from build123d import *

# Parameters (mm, degrees)
BOSS_EXTRUDE10_DEPTH = 1
BOSS_EXTRUDE11_DEPTH = 2
FILLET1_R            = 1
SKETCH22_R           = 1.6
CUT_EXTRUDE1_DEPTH   = 10


with BuildPart() as part:
    # Sketch20 → Boss-Extrude10 (new body)
    with BuildSketch(Plane(origin=(0, 0, 0), x_dir=(1, 0, 0), z_dir=(0, 1, 0))):
        with BuildLine():
            Line((-28, 14.425), (-20.5, 14.425))
            Line((-20.5, 14.425), (-20.5, 13.245))
            Line((-20.5, 13.245), (20.5, 13.245))
            Line((20.5, 13.245), (20.5, 14.425))
            Line((20.5, 14.425), (28, 14.425))
            ThreePointArc((28, 14.425), (28.707106781, 14.132106781), (29, 13.425))
            Line((29, 13.425), (29, -13.425))
            ThreePointArc((29, -13.425), (28.707106781, -14.132106781), (28, -14.425))
            Line((28, -14.425), (20.5, -14.425))
            Line((20.5, -14.425), (20.5, -13.245))
            Line((20.5, -13.245), (-20.5, -13.245))
            Line((-20.5, -13.245), (-20.5, -14.425))
            Line((-20.5, -14.425), (-28, -14.425))
            ThreePointArc((-28, -14.425), (-28.707106781, -14.132106781), (-29, -13.425))
            Line((-29, -13.425), (-29, 13.425))
            ThreePointArc((-29, 13.425), (-28.707106781, 14.132106781), (-28, 14.425))
        make_face()
    extrude(amount=BOSS_EXTRUDE10_DEPTH)

    # Sketch21 → Boss-Extrude11 (add)
    with BuildSketch(Plane.XZ):
        Polygon((-27.825, 3.25), (-26.825, 3.25), (-26.825, -12.25), (16.5, -12.25), (16.5, -13.25), (-27.825, -13.25), align=None)
        Polygon((-17.825, 13.25), (-17.825, 12.25), (26.825, 12.25), (26.825, 0), (27.825, 0), (27.825, 13.25), align=None)
    extrude(amount=BOSS_EXTRUDE11_DEPTH)

    # Fillet1
    fillet1_edges = [part.edges().sort_by_distance(p)[0] for p in [
        (-20.5, 0, -13.8375),
        (20.5, 0, -13.835),
        (20.5, 0, 13.8375),
        (-20.5, 0, 13.835),
    ]]
    fillet(fillet1_edges, radius=FILLET1_R - 0.0001)  # a hair under: the kernel refuses the full size

    # Sketch22 → Cut-Extrude1 (cut)
    with BuildSketch(Plane.XZ):
        with Locations(Location((-24.627459856, 9.750471763, 0), (0, 0, 270))):
            Circle(SKETCH22_R)
    extrude(amount=-CUT_EXTRUDE1_DEPTH, mode=Mode.SUBTRACT)


solid = part.part
Can you work these out from the model? Positions are in its coordinate system, mm. A direction names the side the tool comes from. Give positions to 0.01 mm unless a question says otherwise; leave off trailing zeros. Write each loop counter-clockwise with the first axis right and the second up, starting at its lowest first coordinate (ties: lowest second). Pieces come first, ordered by that corner, then holes. Notation, with made-up numbers: M -20,1.5 L 8,1.5 A29 cw 8,28.5 Z; hole C -12,60.5 d6. An arc over 180 degrees is marked long. Answer in a Markdown table with one row per item. Add a question column.
Item 1: We'd pull the mould along X, two halves only. Please class faces 1 (the flat face through (27.825, -1, 7)), 2 (the flat face through (-12, -2, -13)), 3 (the cylindrical face through (20.801, 0.285, -13.843)): released by +X, released by -X, zero draft, split by the parting line, or undercut.
Item 2: Please list where these lines run through material, in increasing order: L1, parallel to Z at x = -6, y = -0.75; L2, parallel to Y at x = 26, z = -1.75; L3, parallel to Z at x = 24, y = -1.65.
Item 3: Imagine slicing it at A-A, the plane y = -0.9. Write out the boundary of the cut face in (x, z) (3 decimals).
Item 4: Imagine slicing it at C-C, the plane x = -4. Write out the boundary of the cut face in (y, z) (3 decimals).
Item 5: Imagine slicing it at D-D, the plane z = 5.25. Write out the boundary of the cut face in (x, y) (3 decimals), plus the area to 3 significant figures.
Item 6: For pin 1 Ø1 at (x, y) = (-6.5, -0.5) entering from +Z; pin 2 Ø1.6 at (y, z) = (-1, -3.5) entering from -X (3 decimals); pin 3 Ø0.8 at (x, y) = (6, 0.5) entering from -Z (3 decimals), each with a flat end and sliding along its axis, tell me the tip position at first contact or that it passes through.
Item 7: Imagine slicing it at B-B, the plane z = 8.75. Write out the boundary of the cut face in (x, y) (3 decimals).
Item 8: On a 3-axis mill with a long thin cutter (end or side, diameter ignored), from which of +Z, -Z, +X, -X, +Y, -Y can I reach the whole of each face in a straight line? I mean faces 4 (the cylindrical face through (-20.801, 0.285, 13.843)), 5 (the flat face through (-17.825, -1, 13)), 6 (the flat face through (4, -1, 12.25)), 7 (the flat face through (16.5, -1, -13)). Say none if no direction works.
Evaluation:
| question | item | result |
|---|---|---|
| 1 | face 1 | released by +X |
| 1 | face 2 | zero draft |
| 1 | face 3 | undercut |
| 2 | L1 | z = -13.25 to -12.25, 12.25 to 13.25 |
| 2 | L2 | y = 0 to 1 |
| 2 | L3 | z = 12.25 to 13.25 |
| 3 | outline | M -27.825,-13.25 L 16.5,-13.25 L 16.5,-12.25 L -26.825,-12.25 L -26.825,3.25 L -27.825,3.25 Z; M -17.825,12.25 L 26.825,12.25 L 26.825,0 L 27.825,0 L 27.825,13.25 L -17.825,13.25 Z |
| 4 | outline | M -2,-13.25 L 0,-13.25 L 0,-13.245 L 1,-13.245 L 1,13.245 L 0,13.245 L 0,13.25 L -2,13.25 L -2,12.25 L 0,12.25 L 0,-12.25 L -2,-12.25 Z |
| 5 | outline | M -29,0 L 26.825,0 L 26.825,-2 L 27.825,-2 L 27.825,0 L 29,0 L 29,1 L -29,1 Z |
| 5 | area | 60.0 mm² |
| 6 | pin 1 | stops at z = 13.25 |
| 6 | pin 2 | stops at x = -27.825 |
| 6 | pin 3 | stops at z = -13.245 |
| 7 | outline | M -29,0 L -25.876,0 L -25.876,1 L -29,1 Z; M -23.379,0 L 26.825,0 L 26.825,-2 L 27.825,-2 L 27.825,0 L 29,0 L 29,1 L -23.379,1 Z |
| 8 | face 4 | +Z, -Y |
| 8 | face 5 | +Z, -X, -Y |
| 8 | face 6 | -X, -Y |
| 8 | face 7 | -Z, +X, -Y |
